The model under review builds one solid part; all positions refer to its coordinate system, in mm. A direction names the side the tool comes from. Coordinates: 2 decimals unless noted, no trailing zeros. Loops run counter-clockwise (first coordinate to the right, second up) from the corner with the lowest first, then second, coordinate; pieces in that order, holes last. Notation, with made-up numbers: M 6,-37 L 39,-37 A27 ccw 39,-4 Z; hole C 3.5,25.5 d11. An arc over 180 degrees is marked long. Return JSON: item names as keys, results as strings.
```python
from build123d import *

# Parameters (mm, degrees)
SKETCH1_W           = 97
SKETCH1_H           = 149
SKETCH1_R           = 4
BOSS_EXTRUDE1_DEPTH = 6
SKETCH3_W           = 185
SKETCH3_H           = 161
SKETCH3_R           = 3
SKETCH3_R_2         = 3.5
SKETCH3_R_3         = 4
BOSS_EXTRUDE2_DEPTH = 6


with BuildPart() as part:
    # Sketch1 → Boss-Extrude1 (new body)
    with BuildSketch(Plane.XY):
        with Locations((48.5, 74.5)):
            Rectangle(SKETCH1_W, SKETCH1_H)
        with Locations((21, 128)):
            Circle(SKETCH1_R, mode=Mode.SUBTRACT)
        with Locations((75, 128)):
            Circle(SKETCH1_R, mode=Mode.SUBTRACT)
        with Locations((75, 22)):
            Circle(SKETCH1_R, mode=Mode.SUBTRACT)
        with Locations((21, 22)):
            Circle(SKETCH1_R, mode=Mode.SUBTRACT)
    extrude(amount=-BOSS_EXTRUDE1_DEPTH)

    # Sketch3 → Boss-Extrude2 (add)
    with BuildSketch(Plane.XY):
        with Locations((4.5, 80.5)):
            Rectangle(SKETCH3_W, SKETCH3_H)
        with Locations((-77, 155)):
            Circle(SKETCH3_R, mode=Mode.SUBTRACT)
        with Locations((-59, 22)):
            Circle(SKETCH3_R, mode=Mode.SUBTRACT)
        with Locations((-68, 26)):
            Circle(SKETCH3_R_2, mode=Mode.SUBTRACT)
        with Locations((-77, 22)):
            Circle(SKETCH3_R, mode=Mode.SUBTRACT)
        with Locations((-68, 102)):
            Circle(SKETCH3_R_2, mode=Mode.SUBTRACT)
        with Locations((-68, 86)):
            Circle(SKETCH3_R_2, mode=Mode.SUBTRACT)
        with Locations((-68, 65)):
            Circle(SKETCH3_R_2, mode=Mode.SUBTRACT)
        with Locations((-68, 55)):
            Circle(SKETCH3_R_2, mode=Mode.SUBTRACT)
        with Locations((-59, 155)):
            Circle(SKETCH3_R, mode=Mode.SUBTRACT)
        with Locations((-68, 151)):
            Circle(SKETCH3_R_2, mode=Mode.SUBTRACT)
        with Locations((21, 22)):
            Circle(SKETCH3_R_3, mode=Mode.SUBTRACT)
        with Locations((75, 22)):
            Circle(SKETCH3_R_3, mode=Mode.SUBTRACT)
        with Locations((75, 128)):
            Circle(SKETCH3_R_3, mode=Mode.SUBTRACT)
        with Locations((21, 128)):
            Circle(SKETCH3_R_3, mode=Mode.SUBTRACT)
    extrude(amount=BOSS_EXTRUDE2_DEPTH)


solid = part.part
```
1. To check wall thickness, follow line 1 (Y direction, x = -59, z = 1.6); line 2 (Y direction, x = 21, z = 2.5); line 3 (X direction, y = 96, z = -2). State the ranges of each line that lie inside material, in increasing order.
Check values:
{"line 1": "0 to 19, 25 to 152, 158 to 161", "line 2": "0 to 18, 26 to 124, 132 to 161", "line 3": "0 to 97"}
2. Add section C-C on x = -67. Give the boundary of the cut face in (y, z), plus the area to 3 significant figures.
Check values:
{"outline": "M 0,0 L 22.65,0 L 22.65,6 L 0,6 Z; M 29.35,0 L 51.65,0 L 51.65,6 L 29.35,6 Z; M 58.35,0 L 61.65,0 L 61.65,6 L 58.35,6 Z; M 68.35,0 L 82.65,0 L 82.65,6 L 68.35,6 Z; M 89.35,0 L 98.65,0 L 98.65,6 L 89.35,6 Z; M 105.35,0 L 147.65,0 L 147.65,6 L 105.35,6 Z; M 154.35,0 L 161,0 L 161,6 L 154.35,6 Z", "area": "725 mm²"}
3. Machinability: for faces 5 (the face through (-70.58, 57.365, 2.958)), 6 (the face through (48, 76, -6)), 7 (the face through (-38, 82, 0)), 8 (the face through (0, 73, -3)), 9 (the face through (48, 149, -3)), which of the approach directions +Z, -Z, +X, -X, +Y, -Y give a long, thin tool a straight path to every point of the face, cutting with its end or side? Answer none if there is none.
Check values:
{"face 5": "+Z, -Z", "face 6": "-Z, +X, -X, +Y, -Y", "face 7": "-Z, -X, +Y", "face 8": "-Z, -X, +Y, -Y", "face 9": "-Z, +X, -X, +Y"}
4. Add section B-B on z = 2.25. State how many separate pieces and enclosed holes the cut face has, plus the area to 3 significant figures.
Check values:
{"separate pieces": "1", "enclosed holes": "14", "area": "29,200 mm²"}
5. The part is to be moulded in two halves that separate along Y. For faces 1 (the face through (-70.58, 28.365, 2.958)), 2 (the face through (3, 161, 3)), 3 (the face through (97, 79, 0)), 4 (the face through (24, 0, 1)), say which applies: released by +Y, released by -Y, zero draft, split by the parting line, or undercut.
Check values:
{"face 1": "undercut", "face 2": "released by +Y", "face 3": "zero draft", "face 4": "released by -Y"}
6. Add section A-A on x = 21. Give the boundary of the cut face in (y, z).
Check values:
{"outline": "M 0,-6 L 18,-6 L 18,6 L 0,6 Z; M 26,-6 L 124,-6 L 124,6 L 26,6 Z; M 132,-6 L 149,-6 L 149,0 L 161,0 L 161,6 L 132,6 Z"}
7. Add section D-D on y = 49. Give the boundary of the cut face in (x, z), plus the area to 3 significant figures.
Check values:
{"outline": "M -88,0 L 0,0 L 0,-6 L 97,-6 L 97,6 L -88,6 Z", "area": "1,690 mm²"}
8. Insertion check: pin 1 Ø5.5 at (x, y) = (-68, 102) entering from -Z; pin 2 Ø3 at (y, z) = (45.5, -3.5) entering from -X; pin 3 Ø9 at (x, y) = (-68, 65) entering from +Z; pin 4 Ø10 at (x, y) = (-26.5, 120) entering from -Z. Each pin has a flat end and moves straight along its axis. Give the tip position at first contact, or say it passes through.
Check values:
{"pin 1": "through", "pin 2": "x = 0", "pin 3": "z = 6", "pin 4": "z = 0"}
